```python
from build123d import *

# Parameters (mm, degrees)
BOSS_EXTRUDE1_DEPTH      = 4
M5_CLEARANCE_HOLE1_D     = 5.8
FILLET1_R                = 10
M3_CLEARANCE_HOLE1_D     = 3.6
M3_CLEARANCE_HOLE1_DEPTH = 10
M3_CLEARANCE_HOLE1_TIP   = 1.081549114
CHAMFER1_SIZE            = 50
FILLET3_R                = 50
M3_CLEARANCE_HOLE2_D     = 3.6
M3_CLEARANCE_HOLE3_D     = 3.4


with BuildPart() as part:
    # Sketch1 → Boss-Extrude1 (new body)
    with BuildSketch(Plane(origin=(0, 0, 0), x_dir=(1, 0, 0), z_dir=(0, 1, 0))):
        with BuildLine():
            Line((-100, -29.5), (-100, -222))
            Line((-100, -222), (-16, -222))
            Line((-16, -222), (-16, -232))
            Line((-16, -232), (16, -232))
            Line((16, -232), (16, -222))
            Line((16, -222), (100, -222))
            Line((100, -222), (100, -29.5))
            ThreePointArc((100, -29.5), (58, -42.739333694), (16, -29.5))
            Line((16, -29.5), (16, -19.5))
            Line((16, -19.5), (-16, -19.5))
            Line((-16, -19.5), (-16, -29.5))
            ThreePointArc((-16, -29.5), (-58, -42.739333694), (-100, -29.5))
        make_face()
        Polygon((-50.986121811, -69.5), (-5, -69.5), (-5, -100.157414541), align=None, mode=Mode.SUBTRACT)
        Polygon((5, -69.5), (50.986121811, -69.5), (5, -100.157414541), align=None, mode=Mode.SUBTRACT)
        Polygon((60, -75.509252126), (60, -104.5), (16.513878189, -104.5), align=None, mode=Mode.SUBTRACT)
        Polygon((60, -114.5), (60, -143.490747874), (16.513878189, -114.5), align=None, mode=Mode.SUBTRACT)
        Polygon((50.986121811, -149.5), (5, -149.5), (5, -118.842585459), align=None, mode=Mode.SUBTRACT)
        Polygon((-5, -149.5), (-50.986121811, -149.5), (-5, -118.842585459), align=None, mode=Mode.SUBTRACT)
        Polygon((-60, -143.490747874), (-60, -114.5), (-16.513878189, -114.5), align=None, mode=Mode.SUBTRACT)
        Polygon((-16.513878189, -104.5), (-60, -104.5), (-60, -75.509252126), align=None, mode=Mode.SUBTRACT)
    extrude(amount=BOSS_EXTRUDE1_DEPTH)

    # M5 Clearance Hole1 (through all)
    with Locations(Plane(origin=(0, 4, 0), x_dir=(1, 0, 0), z_dir=(0, 1, 0))):
        with Locations((-85, -65), (-85, -145), (85, -145), (85, -65)):
            Hole(M5_CLEARANCE_HOLE1_D / 2)

    # Fillet1
    fillet1_edges = [part.edges().sort_by_distance(p)[0] for p in [
        (100, 2, 29.5),
        (-100, 2, 29.5),
    ]]
    fillet(fillet1_edges, radius=FILLET1_R)

    # M3 Clearance Hole1
    with Locations(Plane(origin=(0, 4, 0), x_dir=(1, 0, 0), z_dir=(0, 1, 0))):
        with Locations((-21, -198), (-21, -180), (20, -180), (20, -198)):
            Hole(M3_CLEARANCE_HOLE1_D / 2, depth=M3_CLEARANCE_HOLE1_DEPTH)
            with Locations((0, 0, -(M3_CLEARANCE_HOLE1_DEPTH + M3_CLEARANCE_HOLE1_TIP / 2))):  # 118° drill point
                Cone(0, M3_CLEARANCE_HOLE1_D / 2, M3_CLEARANCE_HOLE1_TIP, mode=Mode.SUBTRACT)

    # Chamfer1
    chamfer1_edges = [part.edges().sort_by_distance(p)[0] for p in [
        (100, 2, 222),
        (-100, 2, 222),
    ]]
    chamfer(chamfer1_edges, length=CHAMFER1_SIZE)

    # Fillet3
    fillet3_edges = [part.edges().sort_by_distance(p)[0] for p in [
        (100, 2, 172),
        (50, 2, 222),
        (-50, 2, 222),
        (-100, 2, 172),
    ]]
    fillet(fillet3_edges, radius=FILLET3_R)

    # M3 Clearance Hole2 (through all)
    with Locations(Plane(origin=(0, 4, 0), x_dir=(1, 0, 0), z_dir=(0, 1, 0))):
        with Locations((-76, -54.5), (76, -54.5), (76, -161.5), (-76, -161.5), (-10, -24.5), (10, -24.5), (-10, -227), (10, -227)):
            Hole(M3_CLEARANCE_HOLE2_D / 2)

    # M3 Clearance Hole3 (through all)
    with Locations(Plane(origin=(0, 4, 0), x_dir=(1, 0, 0), z_dir=(0, 1, 0))):
        with Locations((53, -180), (34, -180), (34, -205), (53, -205)):
            Hole(M3_CLEARANCE_HOLE3_D / 2)


solid = part.part
```
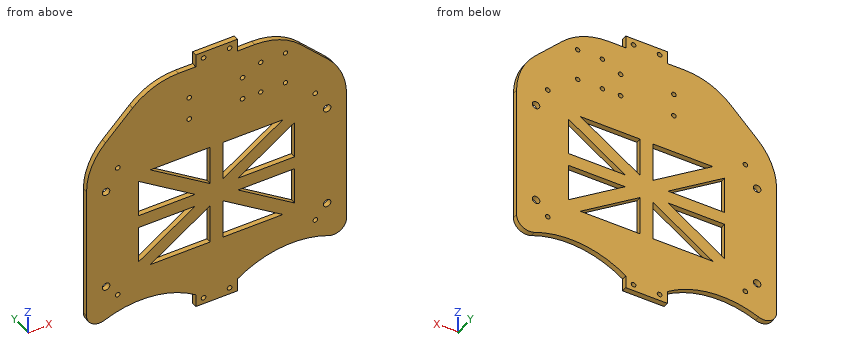
Part model, mm, in its own coordinate system. Give positions to 0.01 mm unless a question says otherwise; leave off trailing zeros. Order: outer loops, then holes, each group sorted by start corner. A loop starts at its lowest first (then second) coordinate and runs counter-clockwise, first axis right, second up. Notation, with made-up numbers: M 14.25,-19 L 57.25,-19 A25 ccw 57.25,4 Z; hole C 65,67.5 d8. An arc over 180 degrees is marked long. Use a Markdown table: item, result. Add a question column.
(1) Probe line 1 along X through (y, z) = (1.5, 24.5); line 2 along X through (y, z) = (1.15, 180); line 3 along X through (y, z) = (1.65, 54.5). List the from-to ranges inside material, lowest first. Write a range as [from, to].
(2) Saw through at A-A, the plane x = -47.5. Give the cut face in (y, z), and give its area (3 significant figures).
(3) Saw through at D-D, the plane z = 166.5. Give the cut face in (x, y).
(4) Drop flat-ended pins along their axis: P1, Ø2, axis at y = 3.5, z = 193, coming from the -X side; P2, Ø1, axis at x = 24, y = 3, coming from the -Z side; P3, Ø1.2, axis at x = -20.5, y = 3, coming from the -Z side. Give the stop position or say it passes through.
(5) Saw through at C-C, the plane z = 219. Give the cut face in (x, y).
(6) Saw through at B-B, the plane y = 2.45. Give the number of separate pieces and of enclosed holes in the cut face, and give its area (3 significant figures).
Answer key:
| question | item | result |
|---|---|---|
| 1 | line 1 | [-16, -11.8], [-8.2, 8.2], [11.8, 16] |
| 1 | line 2 | [-90.94, -22.8], [-19.2, 18.2], [21.8, 32.3], [35.7, 51.3], [54.7, 90.94] |
| 1 | line 3 | [-100, -77.8], [-74.2, 74.2], [77.8, 100] |
| 2 | outline | M 0,41.98 L 4,41.98 L 4,69.5 L 0,69.5 Z; M 0,71.82 L 4,71.82 L 4,83.84 L 0,83.84 Z; M 0,104.5 L 4,104.5 L 4,114.5 L 0,114.5 Z; M 0,135.16 L 4,135.16 L 4,147.18 L 0,147.18 Z; M 0,149.5 L 4,149.5 L 4,218.57 L 0,218.57 Z |
| 2 | area | 522 mm^2 |
| 3 | outline | M -97.63,0 L 97.63,0 L 97.63,4 L -97.63,4 Z |
| 4 | P1 | x = -80 |
| 4 | P2 | z = 34.1 |
| 4 | P3 | z = 32.05 |
| 5 | outline | M -46.35,0 L 46.35,0 L 46.35,4 L -46.35,4 Z |
| 6 | separate pieces | 1 |
| 6 | enclosed holes | 28 |
| 6 | area | 29,200 mm^2 |
